```python
from build123d import *

# Parameters (mm, degrees)
SKETCH2_R          = 2.3876
CUT_EXTRUDE1_DEPTH = 18.161


with BuildPart() as part:
    # Sketch1 → Revolve1 (revolve)
    with BuildSketch(Plane.XY):
        Polygon((0, 0), (9.525, 0), (9.525, -44.45), (7.9375, -44.45), (7.9375, -73.025), (4.7625, -76.2), (0, -76.2), align=None)
    revolve(axis=Axis((0, 76.054523893, 0), (0, -1, 0)))

    # Sketch2 → Cut-Extrude1 (cut, symmetric)
    with BuildSketch(Plane.XY):
        with Locations((0, -8.128)):
            Circle(SKETCH2_R)
        with Locations((0, -14.478)):
            Circle(SKETCH2_R)
        with Locations((0, -20.828)):
            Circle(SKETCH2_R)
        with Locations((0, -27.178)):
            Circle(SKETCH2_R)
        with Locations((0, -33.528)):
            Circle(SKETCH2_R)
    extrude(amount=CUT_EXTRUDE1_DEPTH, both=True, mode=Mode.SUBTRACT)


solid = part.part
```
The listing builds one solid part. Answer for the finished solid, in the listing's coordinates (mm). A direction names the side the tool comes from. Round coordinates to 2 decimals unless told otherwise and drop trailing zeros. Write each loop counter-clockwise with the first axis right and the second up, starting at its lowest first coordinate (ties: lowest second). Pieces come first, ordered by that corner, then holes. Notation, with made-up numbers: (9, -36) -> (58, -36) arc R6 ccw to (58, -29) -> close; hole circle Ø9 at (50, -29). An arc over 180 degrees is marked (long way). Answer as a JSON object with one key per item and string values. Group by question number.
Q1. Which of the six approach directions +Z, -Z, +X, -X, +Y, -Y give full straight-line access (tool end or side, diameter ignored) to faces 1 (the face through (4.4, -22.54, -8.45)), 2 (the face through (-1.72, -58.94, -7.75))?
Q2. Determine the mould class of faces 3 (the face through (1.102, -35.646, 0.133)), 4 (the face through (-1.066, -76.046, -4.8)), 5 (the face through (0, 0, 0)) for opening direction Y: pulls with the +Y half, pulls with the -Y half, needs draft (parallel to the pull), parting line crosses it, or undercut.
Q3. Section A-A (x = 0) is taken. Count the separate pieces of the cut face and the enclosed holes in it, plus the area to 3 significant figures.
Q4. Section B-B (y = -57.5) is taken. Write down the section's boundary in (x, z) (1 decimal).
Q5. Each of these flat-tipped pins is pushed along its axis until it touches: pin 1 Ø3 at (x, y) = (0, -14.478) entering from +Z; pin 2 Ø5 at (x, y) = (3.5, -45.5) entering from +Z; pin 3 Ø5 at (x, y) = (-4.5, -55.5) entering from +Z; pin 4 Ø5 at (y, z) = (-45, -7) entering from -X. Where does it stop, or does it pass through?
Q6. Straight lines are drawn through the part: line 1 along Y through (x, z) = (0, 0); line 2 along Y through (x, z) = (1, 3.5); line 3 along X through (y, z) = (-23, 7.5). For each, find the intervals that lie inside material, in ascending order.
Check values:
{
 "1": {"face 1": "+Y, -Y", "face 2": "-Y"},
 "2": {"face 3": "undercut", "face 4": "pulls with the -Y half", "face 5": "pulls with the +Y half"},
 "3": {"separate pieces": "6", "enclosed holes": "0", "area": "886 mm^2"},
 "4": {"outline": "circle Ø15.9 at (0, 0)"},
 "5": {"pin 1": "through", "pin 2": "z = 9.45", "pin 3": "z = 7.68", "pin 4": "x = -8.36"},
 "6": {"line 1": "-76.2 to -35.92, -31.14 to -29.57, -24.79 to -23.22, -18.44 to -16.87, -12.09 to -10.52, -5.74 to 0", "line 2": "-76.2 to -35.7, -31.36 to -29.35, -25.01 to -23, -18.66 to -16.65, -12.31 to -10.3, -5.96 to 0", "line 3": "-5.87 to -0.99, 0.99 to 5.87"}
}
